```python
from build123d import *

# Parameters (mm, degrees)
SKETCH1_W           = 70
SKETCH1_H           = 40
BOSS_EXTRUDE2_DEPTH = 40
SHELL2_T            = -3
SKETCH2_R           = 3.5
CUT_EXTRUDE1_DEPTH  = 40
SKETCH5_W           = 9
SKETCH5_H           = 15
CUT_EXTRUDE2_DEPTH  = 40
FILLET1_R           = 3


with BuildPart() as part:
    # Sketch1 → Boss-Extrude2 (new body)
    with BuildSketch(Plane.XY):
        Rectangle(SKETCH1_W, SKETCH1_H)
    extrude(amount=BOSS_EXTRUDE2_DEPTH)

    # Shell2
    shell2_openings = [part.faces().sort_by_distance(p)[0] for p in [
        (0, 0, 40),
    ]]
    offset(amount=SHELL2_T, openings=shell2_openings, kind=Kind.INTERSECTION)

    # Sketch2 → Cut-Extrude1 (cut)
    with BuildSketch(Plane(origin=(0, 0, 0), x_dir=(-1, 0, 0), z_dir=(0, 0, -1))):
        Circle(SKETCH2_R)
    extrude(amount=-CUT_EXTRUDE1_DEPTH, mode=Mode.SUBTRACT)

    # Sketch5 → Cut-Extrude2 (cut)
    with BuildSketch(Plane.ZY.offset(35)):
        with Locations((30.5, 0)):
            Rectangle(SKETCH5_W, SKETCH5_H)
    extrude(amount=-CUT_EXTRUDE2_DEPTH, mode=Mode.SUBTRACT)

    # Fillet1
    fillet1_edges = [part.edges().sort_by_distance(p)[0] for p in [
        (35, -20, 20),
        (-35, -20, 20),
        (-35, 20, 20),
        (35, 20, 20),
    ]]
    fillet(fillet1_edges, radius=FILLET1_R)


solid = part.part
```
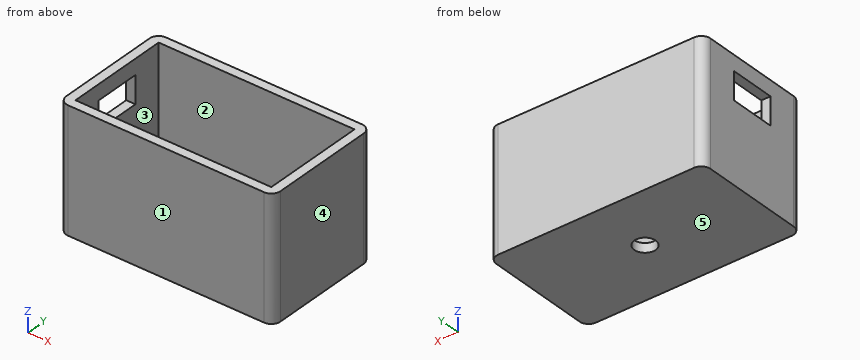
Could you check a few things on this model? Use its own coordinates, in mm. Face numbers are marked on the shaded views. A direction names the side the tool comes from. Round coordinates to 2 decimals unless told otherwise and drop trailing zeros. Loops run counter-clockwise (first coordinate to the right, second up) from the corner with the lowest first, then second, coordinate; pieces in that order, holes last. Notation, with made-up numbers: (3.25, -38) - (41.25, -38) arc R27 cw to (41.25, -21) - close; hole circle Ø1 at (20, 45.25). An arc over 180 degrees is marked (long way). Answer in a Markdown table with one row per item. Add a question column.
(1) I'm going to push a flat-ended pin straight in: pin 1 (5.5 mm diameter, centred on x = 0, y = 0, fed in from +Z). Where does the tip first touch, or does it pass through?
(2) For the marked faces 1 and 2, which set-ups out of +Z, -Z, +X, -X, +Y, -Y let a thin tool reach every point of the face, with its end or its side?
(3) If we mould it in two halves opening along X, with no side actions, what happens to the marked faces 3, 4 and 5? For each: pulls with the +X half, pulls with the -X half, needs draft (parallel to the pull), parting line crosses it, or undercut.
(4) If we section it at D-D (z = 37.5): Please give me the cut outline in (x, y), plus the area to 3 significant figures.
(5) I need wall thicknesses on line 1 along Y through (x, z) = (12, 35.5); line 2 along X through (y, z) = (10, 21); line 3 along Y through (x, z) = (0, 1). Which ranges of each line are inside material? Lowest first, please.
(6) If we section it at C-C (y = 0): Please give me the cut outline in (x, z).
(7) If we section it at B-B (y = -12): Please give me the cut outline in (x, z).
(8) If we section it at A-A (x = 0): Please give me the cut outline in (y, z), plus the area to 3 significant figures.
Model answer:
| question | item | result |
|---|---|---|
| 1 | pin 1 | passes through |
| 2 | face 1 | +Z, -Z, +X, -X, -Y |
| 2 | face 2 | +Z |
| 3 | face 3 | undercut |
| 3 | face 4 | pulls with the +X half |
| 3 | face 5 | needs draft |
| 4 | outline | (-35, -17) arc R3 ccw to (-32, -20) - (32, -20) arc R3 ccw to (35, -17) - (35, 17) arc R3 ccw to (32, 20) - (-32, 20) arc R3 ccw to (-35, 17) - close; hole (-32, -17) - (32, -17) - (32, 17) - (-32, 17) - close |
| 4 | area | 616 mm² |
| 5 | line 1 | y = -20 to -17, 17 to 20 |
| 5 | line 2 | x = -35 to -32, 32 to 35 |
| 5 | line 3 | y = -20 to -3.5, 3.5 to 20 |
| 6 | outline | (-35, 0) - (-3.5, 0) - (-3.5, 3) - (-32, 3) - (-32, 26) - (-35, 26) - close; (-35, 35) - (-32, 35) - (-32, 40) - (-35, 40) - close; (3.5, 0) - (35, 0) - (35, 40) - (32, 40) - (32, 3) - (3.5, 3) - close |
| 7 | outline | (-35, 0) - (35, 0) - (35, 40) - (32, 40) - (32, 3) - (-32, 3) - (-32, 40) - (-35, 40) - close |
| 8 | outline | (-20, 0) - (-3.5, 0) - (-3.5, 3) - (-17, 3) - (-17, 40) - (-20, 40) - close; (3.5, 0) - (20, 0) - (20, 40) - (17, 40) - (17, 3) - (3.5, 3) - close |
| 8 | area | 321 mm² |
